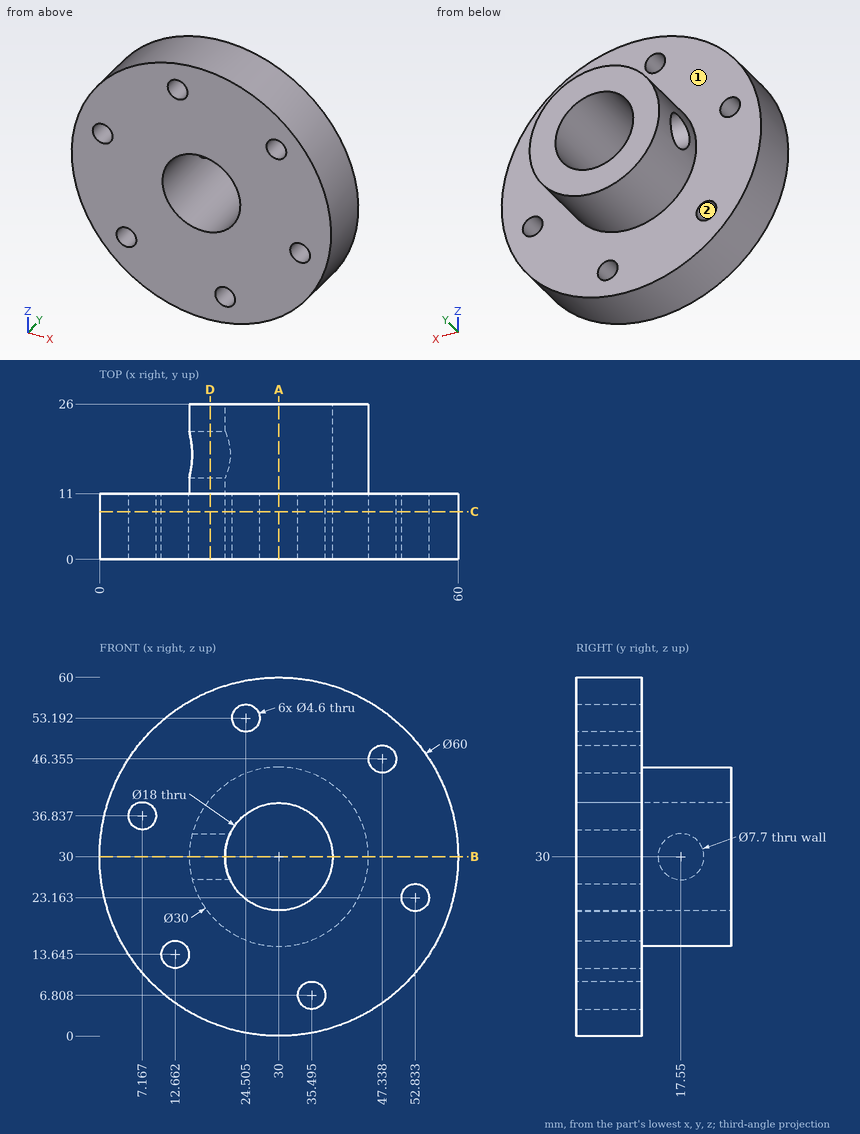
Could you check a few things on this drawing? It's one solid part, dimensions in mm from its lowest x, y, z. A direction names the side the tool comes from. Round coordinates to 2 decimals unless told otherwise and drop trailing zeros. Order: outer loops, then holes, each group sorted by start corner. A loop starts at its lowest first (then second) coordinate and runs counter-clockwise, first axis right, second up.
(1) Please list where these lines run through material, in increasing order: line 1 along X through (y, z) = (7.25, 35.5) (1 decimal); line 2 along Z through (x, y) = (35.5, 10.75) (1 decimal); line 3 along Y through (x, z) = (28, 47).
Response values:
line 1: x = 0.5 to 5.3, 9 to 22.9, 37.1 to 59.5
line 2: z = 0.5 to 4.5, 9.1 to 22.9, 37.1 to 59.5
line 3: y = 0 to 11
(2) Imagine slicing it at A-A (x = 30). Write out the boundary of the cut face in (y, z), plus the area to 3 significant figures.
Response values:
outline: (0, 0) - (11, 0) - (11, 15) - (26, 15) - (26, 21) - (0, 21) - close; (0, 39) - (26, 39) - (26, 45) - (11, 45) - (11, 60) - (0, 60) - close
area: 642 mm2
(3) Imagine slicing it at D-D (x = 18.5). Write out the boundary of the cut face in (y, z), plus the area to 3 significant figures.
Response values:
outline: (0, 2.29) - (11, 2.29) - (11, 20.37) - (26, 20.37) - (26, 39.63) - (11, 39.63) - (11, 57.71) - (0, 57.71) - close; hole circle Ø7.7 at (17.55, 30)
area: 852 mm2
(4) Imagine slicing it at B-B (z = 30). Write out the boundary of the cut face in (x, y), plus the area to 3 significant figures.
Response values:
outline: (0, 0) - (21, 0) - (21, 13.7) - (15, 13.7) - (15, 11) - (0, 11) - close; (15, 21.4) - (21, 21.4) - (21, 26) - (15, 26) - close; (39, 0) - (60, 0) - (60, 11) - (45, 11) - (45, 26) - (39, 26) - close
area: 596 mm2
(5) Imagine slicing it at C-C (y = 8). Write out the boundary of the cut face in (x, z) (1 decimal), plus the area to 3 significant figures.
Response values:
outline: circle Ø60 at (30, 30); hole circle Ø4.6 at (7.2, 36.8); hole circle Ø4.6 at (12.7, 13.6); hole circle Ø18 at (30, 30); hole circle Ø4.6 at (24.5, 53.2); hole circle Ø4.6 at (35.5, 6.8); hole circle Ø4.6 at (47.3, 46.4); hole circle Ø4.6 at (52.8, 23.2)
area: 2,470 mm2
(6) I'm going to push flat-ended pins straight in: pin 1 (5.5 mm diameter, centred on x = 52.83, z = 23.16, fed in from +Y); pin 2 (5 mm diameter, centred on x = 28, z = 23, fed in from -Y); pin 3 (7 mm diameter, centred on y = 17.55, z = 30, fed in from -X); pin 4 (8 mm diameter, centred on x = 37.5, y = 7.5, fed in from -Z) (1 decimal). Where does each tip first touch, or does it pass through?
Response values:
pin 1: stops at y = 11
pin 2: stops at y = 0
pin 3: stops at x = 38.29
pin 4: stops at z = 0.2
(7) Which directions (+Z, -Z, +X, -X, +Y, -Y) give clear straight access to the entire face, cutting with the end or side of a thin tool? Please do the marked faces 1 and 2.
Response values:
face 1: +Y
face 2: +Y, -Y
